Can you work these out from the model? Positions are in its coordinate system, mm. A direction names the side the tool comes from. Round coordinates to 2 decimals unless told otherwise and drop trailing zeros. Order: outer loops, then holes, each group sorted by start corner. A loop starts at its lowest first (then second) coordinate and runs counter-clockwise, first axis right, second up. Notation, with made-up numbers: M 46,82 L 65,82 A33 cw 65,112 Z; hole C 17,66 d4. An arc over 180 degrees is marked long. Answer as a JSON object with one key per item and string values. Group by question number.
from build123d import *

# Parameters (mm, degrees)
BOSS_EXTRUDE1_DEPTH      = 50
BOSS_EXTRUDE1_DEPTH_BACK = 50
SKETCH3_R                = 4
CHAMFER1_SIZE            = 0.56
SKETCH4_R                = 8.463045105
CUT_EXTRUDE1_DEPTH       = 25.4
SKETCH5_R                = 6.629814771
CUT_EXTRUDE2_DEPTH       = 25.4
CUT_EXTRUDE3_START       = -1.47
SKETCH6_R                = 4
SKETCH6_R_2              = 3.6
CUT_EXTRUDE3_DEPTH       = 0.9


with BuildPart() as part:
    # Sketch3 → Boss-Extrude1 (new, two sides: drawn at the far end of the back side and taken through both)
    with BuildSketch(Plane.XY.offset(-BOSS_EXTRUDE1_DEPTH_BACK)):
        Circle(SKETCH3_R)
    extrude(amount=BOSS_EXTRUDE1_DEPTH + BOSS_EXTRUDE1_DEPTH_BACK)

    # Chamfer1
    chamfer1_edges = [part.edges().sort_by_distance(p)[0] for p in [
        (-4, 0, -50),
        (-4, 0, 50),
    ]]
    chamfer(chamfer1_edges, length=CHAMFER1_SIZE)

    # Sketch4 → Cut-Extrude1 (cut)
    with BuildSketch(Plane.XY.offset(50)):
        Circle(SKETCH4_R)
    extrude(amount=-CUT_EXTRUDE1_DEPTH, mode=Mode.SUBTRACT)

    # Sketch5 → Cut-Extrude2 (cut)
    with BuildSketch(Plane(origin=(0, 0, -50), x_dir=(-1, 0, 0), z_dir=(0, 0, -1))):
        Circle(SKETCH5_R)
    extrude(amount=-CUT_EXTRUDE2_DEPTH, mode=Mode.SUBTRACT)

    # Sketch6 → Cut-Extrude3 (cut)
    with BuildSketch(Plane(origin=(0, 0, -24.6), x_dir=(-1, 0, 0), z_dir=(0, 0, -1)).offset(CUT_EXTRUDE3_START)):
        Circle(SKETCH6_R)
        Circle(SKETCH6_R_2, mode=Mode.SUBTRACT)
    cut_extrude3 = extrude(amount=-CUT_EXTRUDE3_DEPTH, mode=Mode.SUBTRACT)

    # Mirror1: Cut-Extrude3 across plane
    add(cut_extrude3.mirror(Plane(origin=(0, 0, 0), x_dir=(1, 0, 0), z_dir=(0, 0, -1))), mode=Mode.SUBTRACT)


solid = part.part
Item 1: I'm going to push a flat-ended pin straight in: pin 1 Ø1 at (x, z) = (-3, -10.5) entering from +Y. Where does the tip first touch, or does it pass through?
Item 2: Suppose I cut it at C-C, the plane z = 21.5. Write out the boundary of the cut face in (x, y).
Item 3: Suppose I cut it at A-A, the plane x = 1.5. Write out the boundary of the cut face in (y, z), and give its area (3 significant figures).
Item 4: I need wall thicknesses on line 1 (Z direction, x = -3.5, y = 1.25); line 2 (X direction, y = 1.75, z = 6.5); line 3 (X direction, y = 2.5, z = 17). Which ranges of each line are inside material? Lowest first, please.
Item 5: Suppose I cut it at B-B, the plane y = 1. Write out the boundary of the cut face in (x, z).
Item 6: On a 3-axis mill with a long thin cutter (end or side, diameter ignored), from which of +Z, -Z, +X, -X, +Y, -Y can I reach the whole of each face in a straight line? I mean faces 1 (the face through (-0.867, -3.905, 23.855)), 2 (the face through (-3.434, 1.081, -22.686)). Say none if no direction works.
Computed:
{
 "1": {"pin 1": "stops at y = 3.12"},
 "2": {"outline": "C 0,0 d8"},
 "3": {"outline": "M -3.71,-24.6 L 3.71,-24.6 L 3.71,-23.13 L 3.27,-23.13 L 3.27,-22.23 L 3.71,-22.23 L 3.71,22.23 L 3.27,22.23 L 3.27,23.13 L 3.71,23.13 L 3.71,24.6 L -3.71,24.6 L -3.71,23.13 L -3.27,23.13 L -3.27,22.23 L -3.71,22.23 L -3.71,-22.23 L -3.27,-22.23 L -3.27,-23.13 L -3.71,-23.13 Z", "area": "363 mm^2"},
 "4": {"line 1": "z = -24.6 to -23.13, -22.23 to 22.23, 23.13 to 24.6", "line 2": "x = -3.6 to 3.6", "line 3": "x = -3.12 to 3.12"},
 "5": {"outline": "M -3.87,-24.6 L 3.87,-24.6 L 3.87,-23.13 L 3.46,-23.13 L 3.46,-22.23 L 3.87,-22.23 L 3.87,22.23 L 3.46,22.23 L 3.46,23.13 L 3.87,23.13 L 3.87,24.6 L -3.87,24.6 L -3.87,23.13 L -3.46,23.13 L -3.46,22.23 L -3.87,22.23 L -3.87,-22.23 L -3.46,-22.23 L -3.46,-23.13 L -3.87,-23.13 Z"},
 "6": {"face 1": "+Z, -Z", "face 2": "none"}
}
